Geometry: final body of the model. Coordinates: model frame, mm. A direction names the side the tool comes from. Give positions to 0.01 mm unless a question says otherwise; leave off trailing zeros. Loops run counter-clockwise (first coordinate to the right, second up) from the corner with the lowest first, then second, coordinate; pieces in that order, holes last. Notation, with made-up numbers: M 7.5,81.25 L 20.5,81.25 A18 cw 20.5,115.25 Z; hole C -7.75,12.25 d6. An arc over 180 degrees is marked long. Put each result on its own line as item: value.
```python
from build123d import *

# Parameters (mm, degrees)
BOSS_EXTRUDE1_DEPTH            = 75
BOSS_EXTRUDE1_DEPTH_BACK       = 75
FILLET1_R                      = 32
FILLET2_R                      = 4
SKETCH2_R                      = 1.55
CUT_EXTRUDE1_DEPTH             = 30
SKETCH3_R                      = 1.55
CUT_EXTRUDE2_DEPTH             = 30
CUT_EXTRUDE4_DEPTH             = 25
CUT_EXTRUDE4_DEPTH_BACK        = 3.4
SKETCH6_R                      = 2.1
CUT_EXTRUDE5_DEPTH             = 84.719770816
CBORE_FOR_M4_SHCS1_D           = 4.5
CBORE_FOR_M4_SHCS1_CBORE_D     = 8
CBORE_FOR_M4_SHCS1_CBORE_DEPTH = 5
BOSS_EXTRUDE2_DEPTH            = 12
CUT_EXTRUDE3_DEPTH             = 25
CUT_EXTRUDE3_DEPTH_BACK        = 3.4
BOSS_EXTRUDE3_START            = -87.5
BOSS_EXTRUDE3_DEPTH            = 12
BOSS_EXTRUDE4_DEPTH            = 12
SKETCH14_W                     = 12
SKETCH14_H                     = 10
CUT_EXTRUDE8_DEPTH             = 84.719770816
SKETCH15_W                     = 6.6
SKETCH15_H                     = 10
SKETCH15_W_2                   = 11
SKETCH15_W_3                   = 15.9
CUT_EXTRUDE9_DEPTH             = 84.719770816
FILLET3_R                      = 1
CHAMFER1_SIZE                  = 4
CHAMFER1_SIZE2                 = 10.989909678


with BuildPart() as part:
    # Sketch1 → Boss-Extrude1 (new, two sides: drawn at the far end of the back side and taken through both)
    with BuildSketch(Plane(origin=(0, 0, 0), x_dir=(0, 0, -1), z_dir=(1, 0, 0)).offset(-BOSS_EXTRUDE1_DEPTH_BACK)):
        with BuildLine():
            Line((-30, -6), (-20, -6))
            Line((-20, -6), (-20, 0.676635828))
            ThreePointArc((-20, 0.676635828), (-19.248641632, 3.583827087), (-17.182746328, 5.762904186))
            Line((-17.182746328, 5.762904186), (-7.4264081, 11.867959502))
            ThreePointArc((-7.4264081, 11.867959502), (0, 14), (7.4264081, 11.867959502))
            Line((7.4264081, 11.867959502), (17.182746328, 5.762904186))
            ThreePointArc((17.182746328, 5.762904186), (19.248641632, 3.583827087), (20, 0.676635828))
            Line((20, 0.676635828), (20, -6))
            Line((20, -6), (30, -6))
            Line((30, -6), (30, 16))
            Line((30, 16), (-30, 16))
            Line((-30, 16), (-30, -6))
        make_face()
    extrude(amount=BOSS_EXTRUDE1_DEPTH + BOSS_EXTRUDE1_DEPTH_BACK)

    # Fillet1
    fillet1_edges = [part.edges().sort_by_distance(p)[0] for p in [
        (-75, 5, 30),
        (75, 5, 30),
    ]]
    fillet(fillet1_edges, radius=FILLET1_R)

    # Fillet2
    fillet2_edges = [part.edges().sort_by_distance(p)[0] for p in [
        (-75, 5, -30),
        (75, 5, -30),
    ]]
    fillet(fillet2_edges, radius=FILLET2_R)

    # Sketch2 → Cut-Extrude1 (cut)
    with BuildSketch(Plane(origin=(0, 0, -30), x_dir=(-1, 0, 0), z_dir=(0, 0, -1))):
        with Locations(Location((36.5, 1.7, 0), (0, 0, 90))):
            Circle(SKETCH2_R)
        with Locations(Location((63.5, 1.7, 0), (0, 0, 90))):
            Circle(SKETCH2_R)
        with Locations(Location((-36.5, 1.7, 0), (0, 0, 90))):
            Circle(SKETCH2_R)
        with Locations(Location((-63.5, 1.7, 0), (0, 0, 90))):
            Circle(SKETCH2_R)
    extrude(amount=-CUT_EXTRUDE1_DEPTH, mode=Mode.SUBTRACT)

    # Sketch3 → Cut-Extrude2 (cut)
    with BuildSketch(Plane.XY.offset(30)):
        with Locations((-13.5, 1.7)):
            Circle(SKETCH3_R)
        with Locations((13.5, 1.7)):
            Circle(SKETCH3_R)
    extrude(amount=-CUT_EXTRUDE2_DEPTH, mode=Mode.SUBTRACT)

    # Sketch5 → Cut-Extrude4 (cut, two sides: drawn at the far end of the back side and taken through both)
    with BuildSketch(Plane(origin=(0, 0, 20), x_dir=(-1, 0, 0), z_dir=(0, 0, -1)).offset(-CUT_EXTRUDE4_DEPTH_BACK)):
        Polygon((-11.91228676, 4.45), (-15.08771324, 4.45), (-16.675426481, 1.7), (-15.08771324, -1.05), (-11.91228676, -1.05), (-10.324573519, 1.7), align=None)
        Polygon((11.91228676, 4.45), (10.324573519, 1.7), (11.91228676, -1.05), (15.08771324, -1.05), (16.675426481, 1.7), (15.08771324, 4.45), align=None)
    extrude(amount=CUT_EXTRUDE4_DEPTH + CUT_EXTRUDE4_DEPTH_BACK, mode=Mode.SUBTRACT)

    # Sketch6 → Cut-Extrude5 (cut, through all)
    with BuildSketch(Plane.XZ.offset(6)):
        with Locations(Location((-20, -25, 0), (0, 0, 270))):
            Circle(SKETCH6_R)
        with Locations(Location((20, -25, 0), (0, 0, 270))):
            Circle(SKETCH6_R)
        with Locations(Location((35, 25, 0), (0, 0, 270))):
            Circle(SKETCH6_R)
        with Locations(Location((-35, 25, 0), (0, 0, 270))):
            Circle(SKETCH6_R)
    extrude(amount=-CUT_EXTRUDE5_DEPTH, mode=Mode.SUBTRACT)

    # CBORE for M4 SHCS1 (through all)
    with Locations(Plane(origin=(0, 16, 0), x_dir=(1, 0, 0), z_dir=(0, 1, 0))):
        with Locations((-20, 25), (20, 25), (35, -25), (-35, -25)):
            CounterBoreHole(CBORE_FOR_M4_SHCS1_D / 2, CBORE_FOR_M4_SHCS1_CBORE_D / 2, CBORE_FOR_M4_SHCS1_CBORE_DEPTH)

    # Sketch12 → Boss-Extrude2 (add)
    with BuildSketch(Plane.ZY.offset(65)):
        with BuildLine():
            Line((20, -6), (13, -6))
            Line((13, -6), (13, 0))
            ThreePointArc((13, 0), (4.088988633, 12.340185248), (-10.427718763, 7.762904186))
            Line((-10.427718763, 7.762904186), (-13.986595688, 7.762904186))
            Line((-13.986595688, 7.762904186), (-7.4264081, 11.867959502))
            ThreePointArc((-7.4264081, 11.867959502), (0, 14), (7.4264081, 11.867959502))
            Line((7.4264081, 11.867959502), (17.182746328, 5.762904186))
            ThreePointArc((17.182746328, 5.762904186), (19.248641632, 3.583827087), (20, 0.676635828))
            Line((20, 0.676635828), (20, -6))
        make_face()
    extrude(amount=-BOSS_EXTRUDE2_DEPTH)

    # Sketch4 → Cut-Extrude3 (cut, two sides: drawn at the far end of the back side and taken through both)
    with BuildSketch(Plane.XY.offset(-20).offset(-CUT_EXTRUDE3_DEPTH_BACK)):
        Polygon((-38.08771324, 4.45), (-39.675426481, 1.7), (-38.08771324, -1.05), (-34.91228676, -1.05), (-33.324573519, 1.7), (-34.91228676, 4.45), align=None)
        Polygon((-65.08771324, 4.45), (-66.675426481, 1.7), (-65.08771324, -1.05), (-61.91228676, -1.05), (-60.324573519, 1.7), (-61.91228676, 4.45), align=None)
        Polygon((34.91228676, 4.45), (33.324573519, 1.7), (34.91228676, -1.05), (38.08771324, -1.05), (39.675426481, 1.7), (38.08771324, 4.45), align=None)
        Polygon((61.91228676, 4.45), (60.324573519, 1.7), (61.91228676, -1.05), (65.08771324, -1.05), (66.675426481, 1.7), (65.08771324, 4.45), align=None)
    extrude(amount=CUT_EXTRUDE3_DEPTH + CUT_EXTRUDE3_DEPTH_BACK, mode=Mode.SUBTRACT)

    # Sketch12<2> → Boss-Extrude3 (add)
    with BuildSketch(Plane.ZY.offset(65).offset(BOSS_EXTRUDE3_START)):
        with BuildLine():
            Line((20, -6), (13, -6))
            Line((13, -6), (13, 0))
            ThreePointArc((13, 0), (4.088988633, 12.340185248), (-10.427718763, 7.762904186))
            Line((-10.427718763, 7.762904186), (-13.986595688, 7.762904186))
            Line((-13.986595688, 7.762904186), (-7.4264081, 11.867959502))
            ThreePointArc((-7.4264081, 11.867959502), (0, 14), (7.4264081, 11.867959502))
            Line((7.4264081, 11.867959502), (17.182746328, 5.762904186))
            ThreePointArc((17.182746328, 5.762904186), (19.248641632, 3.583827087), (20, 0.676635828))
            Line((20, 0.676635828), (20, -6))
        make_face()
    extrude(amount=-BOSS_EXTRUDE3_DEPTH)

    # Sketch13 → Boss-Extrude4 (add)
    with BuildSketch(Plane.ZY.offset(21)):
        with BuildLine():
            Line((-20, -6), (-13, -6))
            Line((-13, -6), (-13, 0))
            ThreePointArc((-13, 0), (-4.088988633, 12.340185248), (10.427718763, 7.762904186))
            Line((10.427718763, 7.762904186), (13.986595688, 7.762904186))
            Line((13.986595688, 7.762904186), (7.4264081, 11.867959502))
            ThreePointArc((7.4264081, 11.867959502), (0, 14), (-7.4264081, 11.867959502))
            Line((-7.4264081, 11.867959502), (-17.182746328, 5.762904186))
            ThreePointArc((-17.182746328, 5.762904186), (-19.248641632, 3.583827087), (-20, 0.676635828))
            Line((-20, 0.676635828), (-20, -6))
        make_face()
    extrude(amount=-BOSS_EXTRUDE4_DEPTH)

    # Sketch14 → Cut-Extrude8 (cut, through all)
    with BuildSketch(Plane(origin=(0, 16, 0), x_dir=(1, 0, 0), z_dir=(0, 1, 0))):
        with Locations((-48.4, 15)):
            Rectangle(SKETCH14_W, SKETCH14_H)
        with Locations((48.4, 15)):
            Rectangle(SKETCH14_W, SKETCH14_H)
        with Locations((0, -15)):
            Rectangle(SKETCH14_W, SKETCH14_H)
    extrude(amount=-CUT_EXTRUDE8_DEPTH, mode=Mode.SUBTRACT)

    # Sketch15 → Cut-Extrude9 (cut, through all)
    with BuildSketch(Plane(origin=(0, 16, 0), x_dir=(1, 0, 0), z_dir=(0, 1, 0))):
        with Locations((-57.7, 15)):
            Rectangle(SKETCH15_W, SKETCH15_H)
        with Locations((-11.5, -15)):
            Rectangle(SKETCH15_W_2, SKETCH15_H)
        with Locations((34.45, 15)):
            Rectangle(SKETCH15_W_3, SKETCH15_H)
    extrude(amount=-CUT_EXTRUDE9_DEPTH, mode=Mode.SUBTRACT)

    # Fillet3
    fillet3_edges = [part.edges().sort_by_distance(p)[0] for p in [
        (30.5, 8.306623863, -10),
        (-13, 8.306623863, 10),
        (-57, 8.306623863, -10),
    ]]
    fillet(fillet3_edges, radius=FILLET3_R)

    # Chamfer1
    chamfer1_edges = [part.edges().sort_by_distance(p)[0] for p in [
        (-51.7, 16, -20),
        (40.45, 16, -20),
        (-5.5, 16, 20),
    ]]
    chamfer1_side = [part.faces().sort_by_distance(p)[0] for p in [
        (-0.052803983, 16, -0.825167589),
    ]]
    chamfer(chamfer1_edges, length=CHAMFER1_SIZE, length2=CHAMFER1_SIZE2, reference=chamfer1_side[0])


solid = part.part
```
Item 1: Set-up query: faces 1 (the cylindrical face through (-34.963, 1.498, -26.746)), 2 (the flat face through (-48, -2, -20)), 3 (the flat face through (-15.89, 3.06, 21.72)), 4 (the cylindrical face through (-59.08, 12.27, 4.3)). Return all of +Z, -Z, +X, -X, +Y, -Y with unobstructed straight access to the full face (end or side cutting, diameter ignored); none if empty.
Output values:
face 1: -Z
face 2: -Y
face 3: none
face 4: +X, -X, -Y
Item 2: Line query: probe 1 along X at (y, z) = (14, -13); probe 2 along X at (y, z) = (14.85, -25); probe 3 along Z at (x, y) = (-20, -0.5). Output: solid intervals per line, ascending. Write a range as [from, to].
Output values:
probe 1: [-75, -61], [-42.4, 26.5], [54.4, 75]
probe 2: [-75, -24], [-16, 16], [24, 75]
probe 3: [-30, -27.25], [-22.75, -13], [20, 30]
Item 3: Section A-A on x = 13.5. Output: boundary loops of the cut face in (y, z), then the cut area to 3 significant figures.
Output values:
outline: M -6,-30 L 16,-30 L 16,30 L 3.25,30 L 3.25,23.4 L 4.45,23.4 L 4.45,18.66 A6 cw 5.76,17.18 L 11.87,7.43 A14 cw 11.87,-7.43 L 5.76,-17.18 A6 cw 0.68,-20 L -6,-20 Z; M -6,20 L -1.05,20 L -1.05,23.4 L 0.15,23.4 L 0.15,30 L -6,30 Z
area: 645 mm²
Item 4: Mould query, pull axis Z, two halves, no side actions, for faces 5 (the cylindrical face through (-21.038, 2.381, -23.004)), 6 (the flat face through (61.13, 3.094, -21.592)), 7 (the cylindrical face through (65.037, 1.498, -26.746)). Classes: pulls with the +Z half, pulls with the -Z half, needs draft (parallel to the pull), parting line crosses it, or undercut.
Output values:
face 5: undercut
face 6: undercut
face 7: needs draft
Item 5: Section D-D on x = 63.5. Output: boundary loops of the cut face in (y, z), then the cut area to 3 significant figures.
Output values:
outline: M -6,-30 L 0.15,-30 L 0.15,-23.4 L -1.05,-23.4 L -1.05,-20 L -6,-20 Z; M -6,20 L 0.68,20 A6 cw 5.76,17.18 L 11.87,7.43 A14 cw 11.87,-7.43 L 5.76,-17.18 A6 cw 4.45,-18.66 L 4.45,-23.4 L 3.25,-23.4 L 3.25,-30 L 16,-30 L 16,22.57 L -6,22.57 Z
area: 482 mm²
Item 6: Section C-C on z = 4. Output: boundary loops of the cut face in (x, y), then the cut area to 3 significant figures.
Output values:
outline: M -74.43,13.42 L -65,13.42 L -65,12.37 L -53,12.37 L -53,13.42 L -21,13.42 L -21,12.37 L -9,12.37 L -9,13.42 L 22.5,13.42 L 22.5,12.37 L 34.5,12.37 L 34.5,13.42 L 74.43,13.42 L 74.43,16 L -74.43,16 Z
area: 422 mm²
Item 7: Section B-B on x = -13.5. Output: boundary loops of the cut face in (y, z), then the cut area to 3 significant figures.
Output values:
outline: M -6,-30 L 16,-30 L 16,10 L 10.72,10 A1 ccw 9.96,8.36 A13 cw 0,-13 L -6,-13 Z; M -6,20 L -1.05,20 L -1.05,23.4 L 0.15,23.4 L 0.15,30 L -6,30 Z; M 3.25,23.4 L 4.45,23.4 L 4.45,20 L 5.01,20 L 16,24 L 16,30 L 3.25,30 Z
area: 651 mm²
Item 8: Pin query (flat end, axial travel): pin 1 Ø4 at (x, y) = (-57.5, 5) entering from +Z; pin 2 Ø6.5 at (x, z) = (18.5, -26) entering from +Y; pin 3 Ø6 at (y, z) = (8, 11) entering from +X; pin 4 Ø6 at (y, z) = (9, -0.5) entering from +X. Return the tip coordinate at first contact, or that it passes through.
Output values:
pin 1: z = 27.46
pin 2: y = 16
pin 3: x = 72.87
pin 4: through
